Could you check a few things on this model? Use its own coordinates, in mm. Give positions to 0.01 mm unless a question says otherwise; leave off trailing zeros. Loops run counter-clockwise (first coordinate to the right, second up) from the corner with the lowest first, then second, coordinate; pieces in that order, holes last. Notation, with made-up numbers: (61.5, -27.75) -> (98.5, -27.75) arc R21 ccw to (98.5, 9.25) -> close; hole circle Ø11 at (56.25, 73.25). An arc over 180 degrees is marked (long way). Write item = value, one per line. Start each with the question number.
1) If we mould it in two halves opening along X, with no side actions, what happens to faces 1 (the face through (30, 1, -17)), 2 (the face through (22.37, 0.61, -36.99)), 3 (the face through (15, 1.2, -23))? For each: +X half, -X half, draft (parallel to the pull), parting line (faces both ways), or undercut.
2) I want a section at A-A (x = 25.75). List the corners of the cut face in (y, z) for me, and give its area (3 significant figures).
3) I want a section at C-C (x = 18.25). List the corners of the cut face in (y, z) for me.
4) I need wall thicknesses on probe 1 along X at (y, z) = (0.55, -22.6); probe 2 along X at (y, z) = (0.5, -2); probe 3 along Z at (x, y) = (15.25, 0.25). Which ranges of each line are inside material? Lowest first, please. Write a range as from..to.
5) I want a section at B-B (y = 0.45). Count the separate pieces of the cut face and the enclosed holes in it, and give its area (3 significant figures).
from build123d import *

# Parameters (mm, degrees)
BOSS_EXTRUDE1_DEPTH = 1.2
CUT_EXTRUDE1_REACH  = 3.2
SKETCH2_R           = 1
SKETCH3_R           = 0.4
CUT_EXTRUDE2_DEPTH  = 1.2
LPATTERN1_COUNT     = 4
LPATTERN1_PITCH     = 9.3
SKETCH4_R           = 0.4
CUT_EXTRUDE3_DEPTH  = 1.2
LPATTERN2_COUNT     = 2
LPATTERN2_PITCH     = 9.3
LPATTERN3_COUNT     = 2
LPATTERN3_PITCH     = 20.5
CUT_EXTRUDE4_REACH  = 3.2
SKETCH5_R           = 0.4


with BuildPart() as part:
    # Sketch1 → Boss-Extrude1 (new body)
    with BuildSketch(Plane(origin=(0, 0, 0), x_dir=(1, 0, 0), z_dir=(0, 1, 0))):
        Polygon((0, 0), (0, 46), (17, 46), (30, 33), (30, 0), align=None)
    extrude(amount=BOSS_EXTRUDE1_DEPTH)

    # Sketch2 → Cut-Extrude1 (cut, up to next)
    with BuildSketch(Plane(origin=(0, 1.2, 0), x_dir=(1, 0, 0), z_dir=(0, 1, 0)), mode=Mode.PRIVATE) as cut_extrude1_sk1:
        with Locations((22.5, 36)):
            Circle(SKETCH2_R)
    cut_extrude1_tool1 = extrude(cut_extrude1_sk1.sketch, amount=-CUT_EXTRUDE1_REACH, mode=Mode.PRIVATE) & part.part
    add(cut_extrude1_tool1.solids().sort_by_distance((22.5, 1.2, -36))[0], mode=Mode.SUBTRACT)

    # Sketch3 → Cut-Extrude2 (cut)
    with BuildSketch(Plane(origin=(0, 1.2, 0), x_dir=(1, 0, 0), z_dir=(0, 1, 0))):
        with Locations((1.5, 2)):
            Circle(SKETCH3_R)
        with Locations((1.5, 4)):
            Circle(SKETCH3_R)
        with Locations((1.5, 6)):
            Circle(SKETCH3_R)
        with Locations((1.5, 8)):
            Circle(SKETCH3_R)
    cut_extrude2 = extrude(amount=-CUT_EXTRUDE2_DEPTH, mode=Mode.SUBTRACT)

    # LPattern1: Cut-Extrude2 ×4
    with Locations(*[(0, 0, -i * LPATTERN1_PITCH) for i in range(1, LPATTERN1_COUNT)]):
        add(cut_extrude2, mode=Mode.SUBTRACT)

    # Sketch4 → Cut-Extrude3 (cut)
    with BuildSketch(Plane(origin=(0, 1.2, 0), x_dir=(1, 0, 0), z_dir=(0, 1, 0))):
        with Locations((28.5, 4.5)):
            Circle(SKETCH4_R)
        with Locations((28.5, 6.5)):
            Circle(SKETCH4_R)
        with Locations((28.5, 8.5)):
            Circle(SKETCH4_R)
        with Locations((28.5, 10.5)):
            Circle(SKETCH4_R)
    cut_extrude3 = extrude(amount=-CUT_EXTRUDE3_DEPTH, mode=Mode.SUBTRACT)

    # LPattern2: Cut-Extrude3 ×2
    with Locations(*[(0, 0, -i * LPATTERN2_PITCH) for i in range(1, LPATTERN2_COUNT)]):
        add(cut_extrude3, mode=Mode.SUBTRACT)

    # LPattern3: Cut-Extrude3 ×2
    with Locations(*[(0, 0, -i * LPATTERN3_PITCH) for i in range(1, LPATTERN3_COUNT)]):
        add(cut_extrude3, mode=Mode.SUBTRACT)

    # Sketch5 → Cut-Extrude4 (cut, up to next)
    with BuildSketch(Plane(origin=(0, 1.2, 0), x_dir=(1, 0, 0), z_dir=(0, 1, 0)), mode=Mode.PRIVATE) as cut_extrude4_sk1:
        with Locations((15.2, 2.2)):
            Circle(SKETCH5_R)
    cut_extrude4_tool1 = extrude(cut_extrude4_sk1.sketch, amount=-CUT_EXTRUDE4_REACH, mode=Mode.PRIVATE) & part.part
    add(cut_extrude4_tool1.solids().sort_by_distance((15.2, 1.2, -2.2))[0], mode=Mode.SUBTRACT)
    # Sketch5 → Cut-Extrude4 (cut, up to next)
    with BuildSketch(Plane(origin=(0, 1.2, 0), x_dir=(1, 0, 0), z_dir=(0, 1, 0)), mode=Mode.PRIVATE) as cut_extrude4_sk2:
        with Locations((17.2, 2.2)):
            Circle(SKETCH5_R)
    cut_extrude4_tool2 = extrude(cut_extrude4_sk2.sketch, amount=-CUT_EXTRUDE4_REACH, mode=Mode.PRIVATE) & part.part
    add(cut_extrude4_tool2.solids().sort_by_distance((17.2, 1.2, -2.2))[0], mode=Mode.SUBTRACT)
    # Sketch5 → Cut-Extrude4 (cut, up to next)
    with BuildSketch(Plane(origin=(0, 1.2, 0), x_dir=(1, 0, 0), z_dir=(0, 1, 0)), mode=Mode.PRIVATE) as cut_extrude4_sk3:
        with Locations((19.2, 2.2)):
            Circle(SKETCH5_R)
    cut_extrude4_tool3 = extrude(cut_extrude4_sk3.sketch, amount=-CUT_EXTRUDE4_REACH, mode=Mode.PRIVATE) & part.part
    add(cut_extrude4_tool3.solids().sort_by_distance((19.2, 1.2, -2.2))[0], mode=Mode.SUBTRACT)
    # Sketch5 → Cut-Extrude4 (cut, up to next)
    with BuildSketch(Plane(origin=(0, 1.2, 0), x_dir=(1, 0, 0), z_dir=(0, 1, 0)), mode=Mode.PRIVATE) as cut_extrude4_sk4:
        with Locations((21.2, 2.2)):
            Circle(SKETCH5_R)
    cut_extrude4_tool4 = extrude(cut_extrude4_sk4.sketch, amount=-CUT_EXTRUDE4_REACH, mode=Mode.PRIVATE) & part.part
    add(cut_extrude4_tool4.solids().sort_by_distance((21.2, 1.2, -2.2))[0], mode=Mode.SUBTRACT)


solid = part.part
Answer list:
q1.face_1 = +X half
q1.face_2 = undercut
q1.face_3 = draft
q2.outline = (0, -37.25) -> (1.2, -37.25) -> (1.2, 0) -> (0, 0) -> close
q2.area = 44.7 mm^2
q3.outline = (0, -44.75) -> (1.2, -44.75) -> (1.2, 0) -> (0, 0) -> close
q4.probe_1 = 0..1.1, 1.9..30
q4.probe_2 = 0..1.1, 1.9..14.85, 15.55..16.85, 17.55..18.85, 19.55..20.85, 21.55..30
q4.probe_3 = -46..-2.6, -1.8..0
q5.separate_pieces = 1
q5.enclosed_holes = 33
q5.area = 1,280 mm^2
